Geometry check sheet. Reference: the model listing, model coordinates, mm. Give positions to 0.01 mm unless a question says otherwise; leave off trailing zeros. Loops run counter-clockwise (first coordinate to the right, second up) from the corner with the lowest first, then second, coordinate; pieces in that order, holes last. Notation, with made-up numbers: (7.25, 26.25) -> (25.25, 26.25) arc R19 ccw to (25.25, 43.25) -> close; hole circle Ø8 at (54.25, 20.25). An arc over 180 degrees is marked (long way). Write each question's results on one line, items separated by ' | '. Start each with the question number.
1) Sectioned sample at B-B on y = -5.5. Record the cut outline in (x, z).
2) Scan lines: line 1 (X direction, y = -7, z = -0.5) (1 decimal); line 2 (Z direction, x = 0, y = -10); line 3 (Y direction, x = 21.5, z = 19). Record each from-to range of solid material in increasing order. Write a range as from..to.
3) Sectioned sample at C-C on y = -26.5. Record the cut outline in (x, z), then the cut area to 3 significant figures.
4) Sectioned sample at D-D on x = 90. Record the cut outline in (y, z), then the cut area to 3 significant figures.
5) Draft check along X on faces 1 (the face through (49.065, -12.325, -20.614)), 2 (the face through (-2.195, -48.125, -9.884)), 3 (the face through (57, -25, 0)). Enter one of: pulls with the +X half, pulls with the -X half, needs draft (parallel to the pull), parting line crosses it, or undercut.
6) Sectioned sample at A-A on x = 0. Record the cut outline in (y, z).
7) Depth check by flat-ended pin: pin 1 (6 mm diameter, centred on x = 13, y = -25.5, fed in from -Z); pin 2 (8 mm diameter, centred on x = 70.5, z = -18, fed in from +Y); pin 3 (8 mm diameter, centred on x = 47, y = -9, fed in from -Z); pin 4 (6 mm diameter, centred on x = 68, z = 15, fed in from -Y). Enter the tip coordinate at first touch or a pass-through.
```python
from build123d import *

# Parameters (mm, degrees)
F0_R     = 10
F1_DEPTH = 25
F2_DEPTH = 50
F3_SIZE  = 2


with BuildPart() as f1:
    # F0 (on Front) → F1 (new body)
    with BuildSketch(Plane.XZ):
        with BuildLine():
            ThreePointArc((7.989306, -23.689048), (20.306805, -14.581964), (25, 0))
            ThreePointArc((25, 0), (20.160232, 14.783946), (7.514795, 23.843822))
            ThreePointArc((7.514795, 23.843822), (-24.998754, -0.249557), (7.989306, -23.689048))
        make_face()
        Circle(F0_R, mode=Mode.SUBTRACT)
        with BuildLine():
            ThreePointArc((7.514795, 23.843822), (20.160232, 14.783946), (25, 0))
            ThreePointArc((25, 0), (20.306805, -14.581964), (7.989306, -23.689048))
            Line((7.989306, -23.689048), (91.306553, -17.451158))
            ThreePointArc((91.306553, -17.451158), (72.500004, 0.01238), (91.331243, 17.449292))
            Line((91.331243, 17.449292), (7.514795, 23.843822))
        make_face()
        with BuildLine():
            ThreePointArc((107.5, 0), (102.836408, 11.894395), (91.331243, 17.449292))
            ThreePointArc((91.331243, 17.449292), (72.500004, 0.01238), (91.306553, -17.451158))
            ThreePointArc((91.306553, -17.451158), (102.82799, -11.903473), (107.5, 0))
        make_face()
        with Locations((90, 0)):
            Circle(F0_R, mode=Mode.SUBTRACT)
    extrude(amount=F1_DEPTH)

    # F0 (on Front) → F2 (join)
    with BuildSketch(Plane.XZ):
        with BuildLine():
            ThreePointArc((7.989306, -23.689048), (20.306805, -14.581964), (25, 0))
            ThreePointArc((25, 0), (20.160232, 14.783946), (7.514795, 23.843822))
            ThreePointArc((7.514795, 23.843822), (-24.998754, -0.249557), (7.989306, -23.689048))
        make_face()
        Circle(F0_R, mode=Mode.SUBTRACT)
    extrude(amount=F2_DEPTH)

    # F3
    f3_edges = [f1.edges().sort_by_distance(p)[0] for p in [
        (-7.989306, -50, 23.689048),
        (-10, -50, 0),
        (80, -25, 0),
    ]]
    chamfer(f3_edges, length=F3_SIZE)


solid = f1.part
```
Result:
1) outline: (7.51, 23.84) arc R25 ccw (long way) to (7.99, -23.69) -> (91.31, -17.45) arc R17.5 ccw to (91.33, 17.45) -> close; hole circle Ø20 at (0, 0); hole circle Ø20 at (90, 0)
2) line 1: -25..-10, 10..80, 100..107.5 | line 2: -25..-10, 10..25 | line 3: -25..0
3) outline: (7.51, 23.84) arc R25 ccw (long way) to (25, 0) arc R25 ccw to start; hole circle Ø20 at (0, 0) | area: 1,650 mm^2
4) outline: (-25, -17.55) -> (0, -17.55) -> (0, -10) -> (-23, -10) -> (-25, -12) -> close; (-25, 12) -> (-23, 10) -> (0, 10) -> (0, 17.55) -> (-25, 17.55) -> close | area: 373 mm^2
5) face 1: pulls with the +X half | face 2: undercut | face 3: needs draft
6) outline: (-50, -23) -> (-48, -25) -> (0, -25) -> (0, -10) -> (-48, -10) -> (-50, -12) -> close; (-50, 12) -> (-48, 10) -> (0, 10) -> (0, 25) -> (-48, 25) -> (-50, 23) -> close
7) pin 1: z = -23.54 | pin 2: y = 0 | pin 3: z = -21.07 | pin 4: y = -25
